```python
from build123d import *

# Parameters (mm, degrees)
ESQUISSE1_R        = 3
ESQUISSE1_R_2      = 3.5
BOSS_EXTRU_1_DEPTH = 1.5


with BuildPart() as part:
    # Esquisse1 → Boss.-Extru.1 (new body)
    with BuildSketch(Plane(origin=(0, 0, 0), x_dir=(1, 0, 0), z_dir=(0, 1, 0))):
        with BuildLine():
            ThreePointArc((4.323150751, -23.607421875), (18.435775248, -15.366267959), (24, 0))
            ThreePointArc((24, 0), (18.435775248, 15.366267959), (4.323150751, 23.607421875))
            ThreePointArc((4.323150751, 23.607421875), (7.562739883, 20.400848266), (8.75, 16))
            ThreePointArc((8.75, 16), (-4.400848266, 8.437260117), (-4.323150751, 23.607421875))
            ThreePointArc((-4.323150751, 23.607421875), (-16.970562748, 16.970562748), (-23.607421875, 4.323150751))
            ThreePointArc((-23.607421875, 4.323150751), (-13.764204997, 8.459534308), (-7.25, 0))
            ThreePointArc((-7.25, 0), (-13.764204997, -8.459534308), (-23.607421875, -4.323150751))
            ThreePointArc((-23.607421875, -4.323150751), (-16.970562748, -16.970562748), (-4.323150751, -23.607421875))
            ThreePointArc((-4.323150751, -23.607421875), (-4.400848266, -8.437260117), (8.75, -16))
            ThreePointArc((8.75, -16), (7.562739883, -20.400848266), (4.323150751, -23.607421875))
        make_face()
        with Locations(Location((-12.542919229, -12.586407821, 0), (0, 0, 270))):
            Circle(ESQUISSE1_R, mode=Mode.SUBTRACT)
        Polygon((11.214276577, -17.821234439), (21, -1.535055726), (22.285750951, -2.307612838), (12.500027528, -18.593791552), align=None, mode=Mode.SUBTRACT)
        with Locations(Location((3, 0, 0), (0, 0, 270))):
            Circle(ESQUISSE1_R_2, mode=Mode.SUBTRACT)
    extrude(amount=BOSS_EXTRU_1_DEPTH)


solid = part.part
```
Part model, mm, in its own coordinate system. A direction names the side the tool comes from. Give positions to 0.01 mm unless a question says otherwise; leave off trailing zeros. Write each loop counter-clockwise with the first axis right and the second up, starting at its lowest first coordinate (ties: lowest second). Pieces come first, ordered by that corner, then holes. Notation, with made-up numbers: (70, 23) -> (90, 23) arc R27 ccw to (90, 57) -> close; hole circle Ø2 at (-30.75, 74). An arc over 180 degrees is marked (long way). Put each result on its own line as item: value. Start each with the question number.
Item 1: Which spindle directions (+Z, -Z, +X, -X, +Y, -Y) get a long thin tool onto all of the face, cutting with end or side? Do faces 4 (the face through (11.866, 0.74, 18.213)), 5 (the face through (5, 0, -6)). Say none if no direction does.
Item 2: Cut at D-D (x = -6). List the corners of the cut face in (y, z), then the cut area to 3 significant figures.
Item 3: Cut at B-B (x = 3). List the corners of the cut face in (y, z), then the cut area to 3 significant figures.
Item 4: Cut at A-A (z = -18). List the corners of the cut face in (x, y), then the cut area to 3 significant figures.
Item 5: Wall check: L1, parallel to X at y = 1.15, z = 5.5; L2, parallel to X at y = 0.95, z = 16; L3, parallel to X at y = 1.3, z = 14. Give the ranges that are in metal, low to high. Write a range as [from, to].
Item 6: Pull direction Z, two halves, no side cores. Call faces 1 (the face through (-17.11, 0.74, 16.83)), 2 (the face through (-13.69, 0.74, 15.36)), 3 (the face through (5, 1.5, -6)): pulls with the +Z half, pulls with the -Z half, needs draft (parallel to the pull), parting line crosses it, or undercut.
Item 7: Cut at C-C (y = 1.05). List the corners of the cut face in (x, z).
Answer list:
1. face 4: +Y, -Y
1. face 5: +Z, -Z, +X, -X, -Y
2. outline: (0, -23.24) -> (1.5, -23.24) -> (1.5, -22.37) -> (0, -22.37) -> close; (0, -9.63) -> (1.5, -9.63) -> (1.5, 9.63) -> (0, 9.63) -> close; (0, 22.37) -> (1.5, 22.37) -> (1.5, 23.24) -> (0, 23.24) -> close
2. area: 31.5 mm2
3. outline: (0, -7.78) -> (1.5, -7.78) -> (1.5, -3.5) -> (0, -3.5) -> close; (0, 3.5) -> (1.5, 3.5) -> (1.5, 7.78) -> (0, 7.78) -> close
3. area: 12.8 mm2
4. outline: (-15.87, 0) -> (-8.52, 0) -> (-8.52, 1.5) -> (-15.87, 1.5) -> close; (8.52, 0) -> (15.87, 0) -> (15.87, 1.5) -> (8.52, 1.5) -> close
4. area: 22.1 mm2
5. L1: x = [-23.36, -22.81], [-9.19, 18.62], [20.37, 23.36]
5. L2: x = [-17.89, -8.75], [8.75, 12.31], [14.06, 17.89]
5. L3: x = [-19.49, -15.19], [-9.9, -8.52], [8.52, 13.51], [15.26, 19.49]
6. face 1: pulls with the +Z half
6. face 2: undercut
6. face 3: needs draft
7. outline: (-23.61, -4.32) arc R24 ccw to (-4.32, -23.61) arc R8.75 cw (long way) to (4.32, -23.61) arc R24 ccw to (4.32, 23.61) arc R8.75 cw (long way) to (-4.32, 23.61) arc R24 ccw to (-23.61, 4.32) arc R8.75 cw (long way) to start; hole circle Ø6 at (-12.54, 12.59); hole circle Ø7 at (3, 0); hole (11.21, 17.82) -> (21, 1.54) -> (22.29, 2.31) -> (12.5, 18.59) -> close
